For this review, take the finished solid that the model builds, in its own axes (mm). A direction names the side the tool comes from. Give positions to 0.01 mm unless a question says otherwise; leave off trailing zeros. Loops run counter-clockwise (first coordinate to the right, second up) from the corner with the lowest first, then second, coordinate; pieces in that order, holes last. Notation, with made-up numbers: (-15.5, -8) - (-5.5, -8) arc R11 ccw to (-5.5, 7) - close; hole circle Ø10 at (37, 1.5). An arc over 180 degrees is marked (long way). Put each result on its own line as item: value.
Autodesk Inventor part; units mm, degrees
ref_plane "РабПлоскость1" through (0, -0.4556, -12.0524) normal (0.711, -0.0009, 0.7032) x (0, 1, 0.0013)
ref_plane "YZ Plane" through (0, 0, 0) normal (1, 0, 0) x (0, 1, 0)
ref_plane "XZ Plane" through (0, 0, 0) normal (0, 1, 0) x (-1, 0, 0)
sketch "Эскиз1" plane through (0, 0, 0) normal (0, 1, 0) x (-1, 0, 0)
  circle A0 centre (0, 0) radius 5
  circle A1 centre (0, 0) radius 2.6
  circle A2 centre (0, 0) radius 11
  circle A3 centre (8, 0) radius 1.55
  circle A4 centre (-8, 0) radius 1.55
  circle A5 centre (0, 8) radius 1.55
  circle A6 centre (0, -8) radius 1.55
  dimension "d0" = 5.2
  dimension "d1" = 10
  dimension "d2" = 22
  dimension "d3" = 3.1
  dimension "d4" = 3.1
  dimension "d5" = 16
  dimension "d6" = 8
  dimension "d7" = 3.1
  dimension "d8" = 3.1
  dimension "d9" = 8
  dimension "d10" = 8
  dimension "d11" = 16
extrude "Выдавливание1" add sketch "Эскиз1" along normal blind 2 contours A2
extrude "Выдавливание2" add sketch "Эскиз1" along normal blind 10 contours A0
sketch "Эскиз2" plane through (0, 0, 0) normal (1, 0, 0) x (0, 1, 0)
  point P0 (0, 0)
  point P1 (-0.4556, -12.0524)
  point P2 (8.9773, -12.0404)
sketch "Эскиз3" plane through (0, 0, 0) normal (0, 0, 1) x (1, 0, 0)
  point P0 (0, 0)
  point P1 (-11.9191, -0.1213)
  point P2 (-11.9191, 9.5232)
ref_plane "РабПлоскость1" through (0, -0.4556, -12.0524) normal (0.711, -0.0009, 0.7032) x (0, 1, 0.0013)
sketch "Эскиз4" plane through (0, -0.4556, -12.0524) normal (0.711, -0.0009, 0.7032) x (0, 1, 0.0013)
  circle A0 centre (6.1565, 8.569) radius 1.5
  point P0 (0.4709, 8.569)
  dimension "d16" = 3
extrude "Выдавливание3" cut sketch "Эскиз4" along normal up to surface
properties part number "Муфта"
1) Wall thickness on line 1 (Z direction, x = 0, y = 1.5); line 2 (Y direction, x = -2, z = 9); line 3 (Z direction, x = 8, y = 0.75): over which ranges is each line inside the solid? List them lowest first.
Geometry check:
line 1: z = -11 to -9.55, -6.45 to -2.6, 2.6 to 6.45, 9.55 to 11
line 2: y = 0 to 2
line 3: z = -7.55 to -1.55, 1.55 to 7.55
2) Draft analysis for pull direction Z (two halves, no side actions). For faces 1 (the face through (1.08, 5.94, 4.88)), 2 (the face through (0, 0, 3)), 3 (the face through (2.063, 4.93, 1.582)), state which applies: pulls with the +Z half, pulls with the -Z half, needs draft (parallel to the pull), parting line crosses it, or undercut.
Geometry check:
face 1: parting line crosses it
face 2: needs draft
face 3: undercut
3) Take a section at D-D on y = 8. State the section outline as (x, z) points, and give its area (3 significant figures).
Geometry check:
outline: circle Ø10 at (0, 0); hole circle Ø5.2 at (0, 0)
area: 57.3 mm²
4) Take a section at A-A on x = 0. State the section outline as (y, z) points.
Geometry check:
outline: (0, -11) - (2, -11) - (2, -9.55) - (0, -9.55) - close; (0, -6.45) - (2, -6.45) - (2, -5) - (10, -5) - (10, -2.6) - (0, -2.6) - close; (0, 2.6) - (10, 2.6) - (10, 5) - (2, 5) - (2, 6.45) - (0, 6.45) - close; (0, 9.55) - (2, 9.55) - (2, 11) - (0, 11) - close
5) Take a section at B-B on z = 2. State the section outline as (x, y) points, and give its area (3 significant figures).
Geometry check:
outline: (-10.82, 0) - (-1.66, 0) - (-1.66, 10) - (-4.58, 10) - (-4.58, 2) - (-10.82, 2) - close; (1.66, 0) - (10.82, 0) - (10.82, 2) - (4.58, 2) - (4.58, 10) - (1.66, 10) - close
area: 83.4 mm²
6) For faces 4 (the face through (6.522, 0.986, -0.466)), 5 (the face through (-2, 2, -5)), list the 3-axis set-ups (+Z, -Z, +X, -X, +Y, -Y) from which the entire face can be reached by the end or side of a thin tool; tool diameter is ignored.
Geometry check:
face 4: +Y, -Y
face 5: +Y
7) Insertion check: pin 1 Ø6 at (y, z) = (2, 7.5) entering from +X; pin 2 Ø4 at (x, z) = (-5, 6) entering from +Y; pin 3 Ø4 at (x, y) = (-2, 6.5) entering from -Z; pin 4 Ø2.5 at (x, z) = (0, -8) entering from +Y. Each pin has a flat end and moves straight along its axis. Give the tip position at first contact, or say it passes through.
Geometry check:
pin 1: stops at x = 10.04
pin 2: stops at y = 2
pin 3: stops at z = -5
pin 4: passes through
8) Take a section at C-C on x = -9. State the section outline as (y, z) points.
Geometry check:
outline: (0, -6.32) - (2, -6.32) - (2, -1.18) - (0, -1.18) - close; (0, 1.18) - (2, 1.18) - (2, 6.32) - (0, 6.32) - close
